```python
from build123d import *

# Parameters (mm, degrees)
LENGTH_DEPTH                            = 880
CUT_EXTRUDE1_REACH                      = 882.407
SKETCH2_R                               = 2.75
CBORE_FOR_M5_HEX_HEAD_BOLT1_D           = 5.5
CBORE_FOR_M5_HEX_HEAD_BOLT1_CBORE_D     = 9.5
CBORE_FOR_M5_HEX_HEAD_BOLT1_CBORE_DEPTH = 3.58
LPATTERN1_COUNT                         = 4
LPATTERN1_PITCH                         = 150
LPATTERN2_COUNT                         = 4
LPATTERN2_PITCH                         = 150


with BuildPart() as part:
    # Sketch1 → Length (new body)
    with BuildSketch(Plane.XY):
        with BuildLine():
            Line((-20, -25), (-5.471687836, -25))
            Line((-5.471687836, -25), (-4.75, -23.75))
            Line((-4.75, -23.75), (4.75, -23.75))
            Line((4.75, -23.75), (5.471687836, -25))
            Line((5.471687836, -25), (20, -25))
            Line((20, -25), (20, -20))
            Line((20, -20), (9.25, -20))
            Line((9.25, -20), (9.25, -13.3))
            Line((9.25, -13.3), (7.521836642, -13.3))
            Line((7.521836642, -13.3), (4, -7.2))
            Line((4, -7.2), (3.487119155, -7.2))
            ThreePointArc((3.487119155, -7.2), (0, -8), (-3.487119155, -7.2))
            Line((-3.487119155, -7.2), (-4, -7.2))
            Line((-4, -7.2), (-7.521836642, -13.3))
            Line((-7.521836642, -13.3), (-9.25, -13.3))
            Line((-9.25, -13.3), (-9.25, -20))
            Line((-9.25, -20), (-20, -20))
            Line((-20, -20), (-20, -25))
        make_face()
    extrude(amount=LENGTH_DEPTH)

    # Sketch2 → Cut-Extrude1 (cut, up to next)
    with BuildSketch(Plane.XZ.offset(25), mode=Mode.PRIVATE) as cut_extrude1_sk1:
        with Locations((-15, 780)):
            Circle(SKETCH2_R)
    cut_extrude1_tool1 = extrude(cut_extrude1_sk1.sketch, amount=-CUT_EXTRUDE1_REACH, mode=Mode.PRIVATE) & part.part
    # Sketch2 → Cut-Extrude1 (cut, up to next)
    with BuildSketch(Plane.XZ.offset(25), mode=Mode.PRIVATE) as cut_extrude1_sk2:
        with Locations((15, 780)):
            Circle(SKETCH2_R)
    cut_extrude1_tool2 = extrude(cut_extrude1_sk2.sketch, amount=-CUT_EXTRUDE1_REACH, mode=Mode.PRIVATE) & part.part
    cut_extrude1_1 = cut_extrude1_tool1.solids().sort_by_distance((-15, -25, 780))[0]
    add(cut_extrude1_1, mode=Mode.SUBTRACT)
    cut_extrude1_2 = cut_extrude1_tool2.solids().sort_by_distance((15, -25, 780))[0]
    add(cut_extrude1_2, mode=Mode.SUBTRACT)
    cut_extrude1 = cut_extrude1_1 + cut_extrude1_2  # Cut-Extrude1 as one shape, for the pattern or mirror that repeats it

    # CBORE for M5 Hex Head Bolt1 (through all)
    with Locations(Plane.XZ.offset(23.75)):
        with Locations((0, 780)):
            cbore_for_m5_hex_head_bolt1 = CounterBoreHole(CBORE_FOR_M5_HEX_HEAD_BOLT1_D / 2, CBORE_FOR_M5_HEX_HEAD_BOLT1_CBORE_D / 2, CBORE_FOR_M5_HEX_HEAD_BOLT1_CBORE_DEPTH)

    # LPattern1: Cut-Extrude1 ×4
    with Locations(*[(0, 0, -i * LPATTERN1_PITCH) for i in range(1, LPATTERN1_COUNT)]):
        add(cut_extrude1, mode=Mode.SUBTRACT)

    # LPattern2: CBORE for M5 Hex Head Bolt1 ×4
    with Locations(*[(0, 0, -i * LPATTERN2_PITCH) for i in range(1, LPATTERN2_COUNT)]):
        add(cbore_for_m5_hex_head_bolt1, mode=Mode.SUBTRACT)


solid = part.part
```
The model under review builds one solid part; all positions refer to its coordinate system, in mm. Round coordinates to 2 decimals unless told otherwise and drop trailing zeros. Order: outer loops, then holes, each group sorted by start corner. A loop starts at its lowest first (then second) coordinate and runs counter-clockwise, first axis right, second up. Notation, with made-up numbers: (49, 30.25) - (79, 30.25) arc R32 ccw to (79, 65.25) - close; hole circle Ø11 at (-12.75, 23). An arc over 180 degrees is marked (long way). Answer in a Markdown table with one row per item.
(1) Clearance check with flat-ended pins moving along their axes: P1, Ø2, axis at x = 13, y = -22, coming from the -Z side; P2, Ø10, axis at y = -13, z = 280, coming from the -X side; P3, Ø5.5, axis at x = -13.5, z = 353.5, coming from the +Y side; P4, Ø3.5, axis at x = 0, z = 480, coming from the -Y side. State where each tip first meets the part, or that it passes through.
Result set:
| item | result |
|---|---|
| P1 | stops at z = 0 |
| P2 | stops at x = -9.25 |
| P3 | stops at y = -20 |
| P4 | passes through |
(2) Take a section at A-A on z = 749.5. Write out the cut boundary in (x, y).
Result set:
| item | result |
|---|---|
| outline | (-20, -25) - (-5.47, -25) - (-4.75, -23.75) - (4.75, -23.75) - (5.47, -25) - (20, -25) - (20, -20) - (9.25, -20) - (9.25, -13.3) - (7.52, -13.3) - (4, -7.2) - (3.49, -7.2) arc R8 cw to (-3.49, -7.2) - (-4, -7.2) - (-7.52, -13.3) - (-9.25, -13.3) - (-9.25, -20) - (-20, -20) - close |
(3) For line 1 (X direction, y = -21.65, z = 330); line 2 (Z direction, x = 0, y = -22.15); line 3 (Z direction, x = -15, y = -21.05), list the stretches that pass through material, from the lowest coordinate up. Write a range as from..to.
Result set:
| item | result |
|---|---|
| line 1 | x = -20..-17.75, -12.25..-4.75, 4.75..12.25, 17.75..20 |
| line 2 | z = 0..325.25, 334.75..475.25, 484.75..625.25, 634.75..775.25, 784.75..880 |
| line 3 | z = 0..327.25, 332.75..477.25, 482.75..627.25, 632.75..777.25, 782.75..880 |
